Can you work these out from the model? Positions are in its coordinate system, mm. Round coordinates to 2 decimals unless told otherwise and drop trailing zeros. Order: outer loops, then holes, each group sorted by start corner. A loop starts at its lowest first (then second) coordinate and runs counter-clockwise, first axis right, second up. Notation, with made-up numbers: (68, -28) -> (89, -28) arc R21 ccw to (89, -15) -> close; hole circle Ø4 at (9, 25.5). An arc over 180 degrees is marked (long way). Use a Markdown table: item, result. Add a question column.
Q1. If we section it at C-C on y = 4.25: List the corners of the cut face in (x, z) for me.
Q2. I need wall thicknesses on line 1 along Z through (x, y) = (0, 3.75); line 2 along X through (y, z) = (4, 1). Which ranges of each line are inside material? Lowest first, please. Write a range as [from, to].
Q3. We'd pull the mould along X, two halves only. Please class faces 1 (the face through (-7.25, 3.45, -0.08)), 2 (the face through (13, 0, 0)), 3 (the face through (15.594, 2.465, -5.974)): +X half, -X half, draft (parallel to the pull), parting line (faces both ways), or undercut.
Q4. If we section it at D-D on z = 2.25: List the corners of the cut face in (x, y) for me, plus the area to 3 significant figures.
Q5. If we section it at B-B on x = 5.5: List the corners of the cut face in (y, z) for me, plus the area to 3 significant figures.
Q6. If we section it at A-A on z = -4.5: List the corners of the cut face in (x, y) for me.
Q7. I'm going to push flat-ended pins straight in: pin 1 Ø3 at (x, z) = (0, 5.5) entering from -Y; pin 2 Ø3 at (x, y) = (9.5, 6) entering from -Z; pin 3 Ø5 at (x, z) = (18, 4) entering from +Y; pin 4 Ø4 at (x, y) = (17, 4.5) entering from -Z. Where does each tip first touch, or does it pass through?
```python
from build123d import *

# Parameters (mm, degrees)
SKETCH1_R           = 1.5
SKETCH1_R_2         = 1.75
BOSS_EXTRUDE1_DEPTH = 5
SKETCH2_R           = 8
SKETCH2_R_2         = 1.75
BOSS_EXTRUDE2_DEPTH = 2


with BuildPart() as part:
    # Sketch1 → Boss-Extrude1 (new body)
    with BuildSketch(Plane(origin=(0, 0, 0), x_dir=(1, 0, 0), z_dir=(0, 1, 0))):
        with BuildLine():
            Line((1.066666667, 7.928569999), (30.533333333, 3.964284999))
            ThreePointArc((30.533333333, 3.964284999), (34, 0), (30.533333333, -3.964284999))
            Line((30.533333333, -3.964284999), (1.066666667, -7.928569999))
            ThreePointArc((1.066666667, -7.928569999), (-8, 0), (1.066666667, 7.928569999))
        make_face()
        with Locations((30, 0)):
            Circle(SKETCH1_R, mode=Mode.SUBTRACT)
        with Locations((-5.5, 0)):
            Circle(SKETCH1_R_2, mode=Mode.SUBTRACT)
        with Locations((0, 5.5)):
            Circle(SKETCH1_R_2, mode=Mode.SUBTRACT)
        with Locations((5.5, 0)):
            Circle(SKETCH1_R_2, mode=Mode.SUBTRACT)
        with Locations((0, -5.5)):
            Circle(SKETCH1_R_2, mode=Mode.SUBTRACT)
    extrude(amount=BOSS_EXTRUDE1_DEPTH)

    # Sketch2 → Boss-Extrude2 (add)
    with BuildSketch(Plane(origin=(0, 5, 0), x_dir=(1, 0, 0), z_dir=(0, 1, 0))):
        Circle(SKETCH2_R)
        with Locations((-5.5, 0)):
            Circle(SKETCH2_R_2, mode=Mode.SUBTRACT)
        with Locations((0, -5.5)):
            Circle(SKETCH2_R_2, mode=Mode.SUBTRACT)
        with Locations((5.5, 0)):
            Circle(SKETCH2_R_2, mode=Mode.SUBTRACT)
        with Locations((0, 5.5)):
            Circle(SKETCH2_R_2, mode=Mode.SUBTRACT)
    extrude(amount=BOSS_EXTRUDE2_DEPTH)


solid = part.part
```
Answer below:
| question | item | result |
|---|---|---|
| 1 | outline | (1.07, -7.93) -> (30.53, -3.96) arc R4 ccw to (30.53, 3.96) -> (1.07, 7.93) arc R8 ccw (long way) to start; hole circle Ø3.5 at (-5.5, 0); hole circle Ø3.5 at (0, -5.5); hole circle Ø3.5 at (0, 5.5); hole circle Ø3.5 at (5.5, 0); hole circle Ø3 at (30, 0) |
| 2 | line 1 | [-8, -7.25], [-3.75, 3.75], [7.25, 8] |
| 2 | line 2 | [-7.94, -6.94], [-4.06, 4.06], [6.94, 28.88], [31.12, 33.87] |
| 3 | face 1 | undercut |
| 3 | face 2 | draft |
| 3 | face 3 | +X half |
| 4 | outline | (-7.68, 0) -> (33.31, 0) -> (33.31, 5) -> (7.68, 5) -> (7.68, 7) -> (-7.68, 7) -> close |
| 4 | area | 236 mm² |
| 5 | outline | (0, -7.33) -> (5, -7.33) -> (5, -5.81) -> (7, -5.81) -> (7, -1.75) -> (0, -1.75) -> close; (0, 1.75) -> (7, 1.75) -> (7, 5.81) -> (5, 5.81) -> (5, 7.33) -> (0, 7.33) -> close |
| 5 | area | 72.1 mm² |
| 6 | outline | (-6.61, 0) -> (-1.44, 0) -> (-1.44, 7) -> (-6.61, 7) -> close; (1.44, 0) -> (26.55, 0) -> (26.55, 5) -> (6.61, 5) -> (6.61, 7) -> (1.44, 7) -> close |
| 7 | pin 1 | through |
| 7 | pin 2 | z = -6.94 |
| 7 | pin 3 | y = 5 |
| 7 | pin 4 | z = -6.05 |
